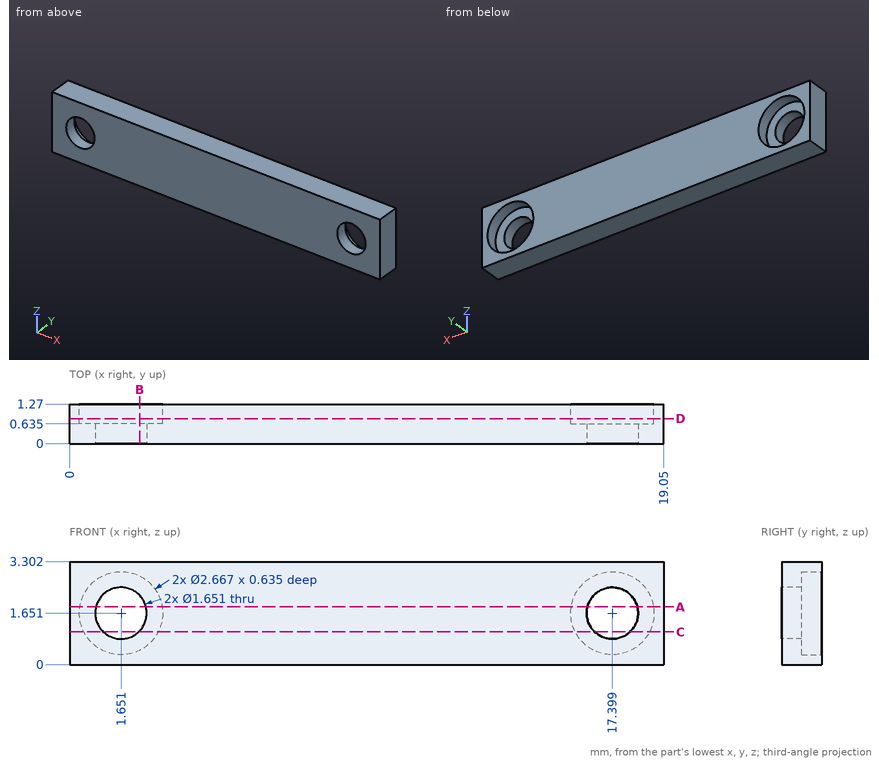
The figure shows three views and two pictorial views of one solid part (mm, origin at its lowest corner). Answer the questions. Round coordinates to 2 decimals unless told otherwise and drop trailing zeros. Order: outer loops, then holes, each group sorted by start corner. A loop starts at its lowest first (then second) coordinate and runs counter-clockwise, first axis right, second up.
Q1. Given pin 1 Ø1 at (x, z) = (1.651, 1.651) entering from -Y, flat-ended and moving along its own axis, determine where the tip first touches the part or whether it passes through.
Solution:
pin 1: passes through
Q2. A cutting plane is placed at B-B, the plane x = 2.25. Determine the outline of the cut face in (y, z) (3 decimals), then the cut area to 3 significant figures.
Solution:
outline: (0, 0) - (1.27, 0) - (1.27, 0.46) - (0.635, 0.46) - (0.635, 1.083) - (0, 1.083) - close; (0, 2.219) - (0.635, 2.219) - (0.635, 2.842) - (1.27, 2.842) - (1.27, 3.302) - (0, 3.302) - close
area: 1.96 mm2
Q3. A cutting plane is placed at C-C, the plane z = 1.05. Determine the outline of the cut face in (x, y) (3 decimals), then the cut area to 3 significant figures.
Solution:
outline: (0, 0) - (1.085, 0) - (1.085, 0.635) - (0.461, 0.635) - (0.461, 1.27) - (0, 1.27) - close; (2.217, 0) - (16.833, 0) - (16.833, 0.635) - (16.209, 0.635) - (16.209, 1.27) - (2.841, 1.27) - (2.841, 0.635) - (2.217, 0.635) - close; (17.965, 0) - (19.05, 0) - (19.05, 1.27) - (18.589, 1.27) - (18.589, 0.635) - (17.965, 0.635) - close
area: 19.7 mm2
Q4. A cutting plane is placed at D-D, the plane y = 0.8. Determine the outline of the cut face in (x, z), then the cut area to 3 significant figures.
Solution:
outline: (0, 0) - (19.05, 0) - (19.05, 3.3) - (0, 3.3) - close; hole circle Ø2.67 at (1.65, 1.65); hole circle Ø2.67 at (17.4, 1.65)
area: 51.7 mm2
Q5. A cutting plane is placed at A-A, the plane z = 1.85. Determine the outline of the cut face in (x, y) (3 decimals), then the cut area to 3 significant figures.
Solution:
outline: (0, 0) - (0.85, 0) - (0.85, 0.635) - (0.332, 0.635) - (0.332, 1.27) - (0, 1.27) - close; (2.452, 0) - (16.598, 0) - (16.598, 0.635) - (16.08, 0.635) - (16.08, 1.27) - (2.97, 1.27) - (2.97, 0.635) - (2.452, 0.635) - close; (18.2, 0) - (19.05, 0) - (19.05, 1.27) - (18.718, 1.27) - (18.718, 0.635) - (18.2, 0.635) - close
area: 18.8 mm2
Q6. Find the intervals of material crossed by line 1 along X through (y, z) = (0.45, 1.65); line 2 along X through (y, z) = (0.95, 2.65); line 3 along Z through (x, y) = (2.25, 1.15), in increasing order.
Solution:
line 1: x = 0 to 0.83, 2.48 to 16.57, 18.22 to 19.05
line 2: x = 0 to 0.77, 2.53 to 16.52, 18.28 to 19.05
line 3: z = 0 to 0.46, 2.84 to 3.3
